```python
from build123d import *

# Parameters (mm, degrees)
F0_W      = 60
F0_H      = 10
F1_DEPTH  = 5
F4_DEPTH  = 5
F6_DEPTH  = 5
F7_DEPTH  = 5
F9_D      = 3
F11_R     = 1
F13_D     = 3
F13_DEPTH = 4
F13_TIP   = 0.9012909285
F14_ANGLE = -90


with BuildPart() as f1:
    # F0 (on Right) → F1 (new body)
    with BuildSketch(Plane.YZ):
        with Locations((30, 10.0670714118)):
            Rectangle(F0_W, F0_H)
    extrude(amount=-F1_DEPTH)

    # F2: F1 across plane


with BuildPart() as f1_1:
    add(f1.part)
    add(f1.part.mirror(Plane.XZ))

    # F3 (on Right) → F4 (join)
    with BuildSketch(Plane.YZ):
        Polygon((-60, 25.0670714118), (-60, 15.0670714118), (-42, 15.0670714118), (-57, 25.0670714118), align=None)
    extrude(amount=-F4_DEPTH)

    # F9 (through all)
    with Locations(Plane.YZ):
        with Locations((0, 10.2355619892)):
            Hole(F9_D / 2)


with BuildPart() as f6:
    # F5 (on face) → F6 (new body)
    with BuildSketch(Plane.YZ):
        Polygon((57, 0), (60, 0), (60, 10.0670714118), (45, 10.0670714118), align=None)
    extrude(amount=F6_DEPTH)


with BuildPart() as f7:
    # F5 (on face) → F7 (new body)
    with BuildSketch(Plane.YZ):
        Polygon((57, 0), (60, 0), (60, 10.0670714118), (45, 10.0670714118), align=None)
    extrude(amount=-F7_DEPTH)


with BuildPart() as f1_2:
    add(f1_1.part)

    # F10: union F6, F7
    add(f6.part)
    add(f7.part)

    # F11
    f11_edges = [f1_2.edges().sort_by_distance(p)[0] for p in [
        (0, 57, 0),
        (0, 60, 0),
    ]]
    fillet(f11_edges, radius=F11_R)

    # F13
    with Locations(Plane(origin=(0, 0, 5.0670714118), x_dir=(1, 0, 0), z_dir=(0, 0, -1))):
        with Locations((-2.6265240659, 45.0005336208)):
            Hole(F13_D / 2, depth=F13_DEPTH)
            with Locations((0, 0, -(F13_DEPTH + F13_TIP / 2))):  # 118° drill point
                Cone(0, F13_D / 2, F13_TIP, mode=Mode.SUBTRACT)


with BuildPart() as f1_3:
    # F14: moved
    add(f1_2.part.rotate(Axis((0, 9, 15.0670714118), (0, 1, 0)), F14_ANGLE))


solid = f1_3.part
```
Work out the finished part from the listing and answer in its coordinate system (mm). A direction names the side the tool comes from. Give positions to 0.01 mm unless a question says otherwise; leave off trailing zeros. Write each loop counter-clockwise with the first axis right and the second up, starting at its lowest first coordinate (ties: lowest second). Pieces come first, ordered by that corner, then holes.
(1) The part is cut by section B-B on z = 18. Write down the section's boundary in (x, y), plus the area to 3 significant figures.
Final values:
outline: (5, 45) - (14.83, 56.72) arc R1 ccw to (15.07, 57.36) - (15.07, 59) arc R1 ccw to (14.07, 60) - (5, 60) - close
area: 90.4 mm2
(2) The part is cut by section A-A on y = 0. Write down the section's boundary in (x, z), plus the area to 3 significant figures.
Final values:
outline: (0, 10.07) - (3.33, 10.07) - (3.33, 15.07) - (0, 15.07) - close; (6.33, 10.07) - (10, 10.07) - (10, 15.07) - (6.33, 15.07) - close
area: 35.0 mm2
(3) The mould has two halves that part along Z. Classify faces 4 (the cylindrical face through (7.97, -43.67, 11.75)), 5 (the conical face through (5.255, -44.746, 12.384)), 6 (the flat face through (-10, -58, 13)), 7 (the flat face through (9, 54, 20.067)): pulls with the +Z half, pulls with the -Z half, needs draft (parallel to the pull), parting line crosses it, or undercut.
Final values:
face 4: undercut
face 5: undercut
face 6: needs draft
face 7: pulls with the +Z half
(4) The part is cut by section D-D on y = -37. Write down the section's boundary in (x, z).
Final values:
outline: (0, 10.07) - (10, 10.07) - (10, 15.07) - (0, 15.07) - close
(5) Which of the six approach directions +Z, -Z, +X, -X, +Y, -Y give full straight-line access (tool end or side, diameter ignored) to faces 1 (the flat face through (10.94, 52.08, 16.25)), 2 (the flat face through (0, 10, 13)), 3 (the flat face through (5, 53, 18))?
Final values:
face 1: +Z, +X, -Y
face 2: +Z, -Z, -X, +Y
face 3: +Z, -X, +Y, -Y
(6) The part is cut by section C-C on x = -8. Write down the section's boundary in (y, z), plus the area to 3 significant figures.
Final values:
outline: (-60, 10.07) - (-54, 10.07) - (-54, 15.07) - (-60, 15.07) - close
area: 30.0 mm2
(7) Straight lines are drawn through the part: line 1 (X direction, y = 0, z = 13.9); line 2 (X direction, y = 3, z = 10.5); line 3 (Y direction, x = 5, z = 14.75). For each, find the intervals that lie inside material, in ascending order.
Final values:
line 1: x = 0 to 3.33, 6.33 to 10
line 2: x = 0 to 10
line 3: y = -60 to -1.49, 1.49 to 60
(8) Flat-ended cylindrical pins translate along their axes: pin 1 Ø4 at (y, z) = (29, 13) entering from -X; pin 2 Ø8 at (x, y) = (-4.5, -44.5) entering from +Z; pin 3 Ø1.5 at (x, z) = (-7.5, 14) entering from +Y (3 decimals); pin 4 Ø10 at (x, y) = (-6, -0.5) entering from -Z. Find the tip coordinate at first contact, or state that the pin passes through.
Final values:
pin 1: stops at x = 0
pin 2: stops at z = 15.07
pin 3: stops at y = -52.125
pin 4: passes through
